The model under review builds one solid part; all positions refer to its coordinate system, in mm. Round coordinates to 2 decimals unless told otherwise and drop trailing zeros. Loops run counter-clockwise (first coordinate to the right, second up) from the corner with the lowest first, then second, coordinate; pieces in that order, holes last. Notation, with made-up numbers: (40.25, 65.5) -> (48.25, 65.5) arc R27 cw to (48.25, 102.5) -> close; hole circle Ø8 at (22.25, 44). An arc over 180 degrees is marked (long way). Use a Markdown table: item, result. Add a question column.
1) Insertion check: pin 1 (1 mm diameter, centred on x = 5, z = -1.5, fed in from -Y); pin 2 (2.5 mm diameter, centred on x = 0, z = 0.5, fed in from -Y); pin 3 (4 mm diameter, centred on x = 1, z = 6, fed in from +Y); pin 4 (1 mm diameter, centred on y = 2, z = -1, fed in from +X). Each pin has a flat end and moves straight along its axis. Give the tip position at first contact, or say it passes through.
2) Consider section A-A on x = -6.5. Give the boundary of the cut face in (y, z), plus the area to 3 significant figures.
3) Wall thickness on probe 1 along Z at (x, y) = (0, 0.8); probe 2 along Z at (x, y) = (0, 1.7); probe 3 along X at (y, z) = (0.6, 0.5): over which ranges is each line inside the solid? List them lowest first.
4) Consider section B-B on y = 2.3. Give the boundary of the cut face in (x, z), plus the area to 3 significant figures.
5) Consider section C-C on z = -6. Give the boundary of the cut face in (x, y).
6) Consider section D-D on x = 0. State how many separate pieces and enclosed holes the cut face has, plus the area to 3 significant figures.
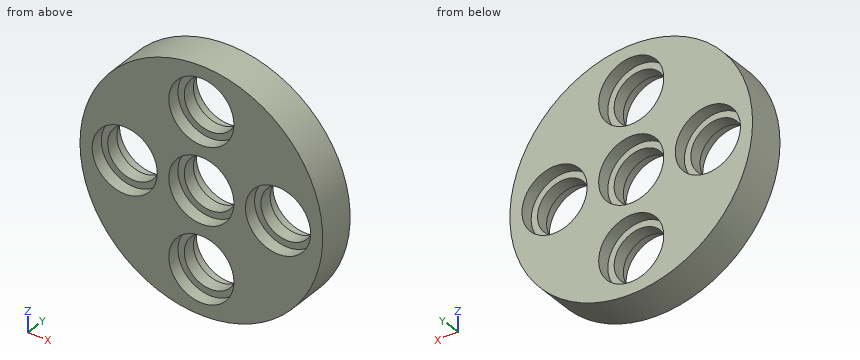
Autodesk Inventor part; units mm, degrees
ref_plane "Work Plane1" through (0, 1.5, 0) normal (0, -1, 0) x (1, 0, 0)
ref_plane "YZ Plane" through (0, 0, 0) normal (1, 0, 0) x (0, 1, 0)
ref_plane "XZ Plane" through (0, 0, 0) normal (0, 1, 0) x (-1, 0, 0)
sketch "Esquisse1" plane through (0, 0, 0) normal (0, 1, 0) x (-1, 0, 0)
  circle A0 centre (0, 0) radius 9.5
  circle A1 centre (0, 0) radius 2.05
  line L0 (0, 9.5) -> (0, -9.5) construction
  line L1 (-9.5, 0) -> (9.5, 0) construction
  circle A2 centre (0, -6) radius 2.05
  circle A3 centre (0, 6) radius 2.05
  circle A4 centre (0, 0) radius 2.05
  circle A5 centre (6, 0) radius 2.05
  circle A6 centre (-6, 0) radius 2.05
  circle A7 centre (0, 0) radius 2.05
  dimension "d0" = 19
  dimension "d1" = 4.1
  dimension "d4" = 6
  dimension "d7" = 6
  dimension "d12" = 6
  dimension "d15" = 6
extrude "Extrusion1" add sketch "Esquisse1" along normal blind 3
sketch "Sketch2" plane through (0, 0, 0) normal (0, -1, 0) x (1, 0, 0)
  circle A0 centre (-6, 0) radius 2.05
  circle A1 centre (-6, 0) radius 2.55
  circle A2 centre (0, 6) radius 2.05
  circle A3 centre (0, 6) radius 2.55
  circle A4 centre (0, 0) radius 2.55
  circle A5 centre (6, 0) radius 2.05
  circle A6 centre (6, 0) radius 2.55
  circle A7 centre (0, -6) radius 2.05
  circle A8 centre (0, -6) radius 2.55
  dimension "d20" = 5.1
  dimension "d21" = 5.1
  dimension "d22" = 5.1
  dimension "d23" = 5.1
  dimension "d24" = 5.1
extrude "Extrusion2" cut sketch "Sketch2" against normal blind 1
ref_plane "Work Plane1" through (0, 1.5, 0) normal (0, -1, 0) x (1, 0, 0)
mirror "Mirror1" about plane through (0, 1.5, 0) normal (0, -1, 0) of "Extrusion2"
properties part number "XL320_IdlerToOllo"
Result set:
| question | item | result |
|---|---|---|
| 1 | pin 1 | y = 1 |
| 1 | pin 2 | through |
| 1 | pin 3 | y = 3 |
| 1 | pin 4 | x = 9.49 |
| 2 | outline | (0, -6.93) -> (3, -6.93) -> (3, -2.5) -> (2, -2.5) -> (2, -1.99) -> (1, -1.99) -> (1, -2.5) -> (0, -2.5) -> close; (0, 2.5) -> (1, 2.5) -> (1, 1.99) -> (2, 1.99) -> (2, 2.5) -> (3, 2.5) -> (3, 6.93) -> (0, 6.93) -> close |
| 2 | area | 27.6 mm2 |
| 3 | probe 1 | -9.5 to -8.55, -3.45 to -2.55, 2.55 to 3.45, 8.55 to 9.5 |
| 3 | probe 2 | -9.5 to -8.05, -3.95 to -2.05, 2.05 to 3.95, 8.05 to 9.5 |
| 3 | probe 3 | -9.49 to -8.5, -3.5 to -2.5, 2.5 to 3.5, 8.5 to 9.49 |
| 4 | outline | circle Ø19 at (0, 0); hole circle Ø5.1 at (-6, 0); hole circle Ø5.1 at (0, -6); hole circle Ø5.1 at (0, 0); hole circle Ø5.1 at (0, 6); hole circle Ø5.1 at (6, 0) |
| 4 | area | 181 mm2 |
| 5 | outline | (-7.37, 0) -> (-2.55, 0) -> (-2.55, 1) -> (-2.05, 1) -> (-2.05, 2) -> (-2.55, 2) -> (-2.55, 3) -> (-7.37, 3) -> close; (2.05, 1) -> (2.55, 1) -> (2.55, 0) -> (7.37, 0) -> (7.37, 3) -> (2.55, 3) -> (2.55, 2) -> (2.05, 2) -> close |
| 6 | separate pieces | 4 |
| 6 | enclosed holes | 0 |
| 6 | area | 14.1 mm2 |
